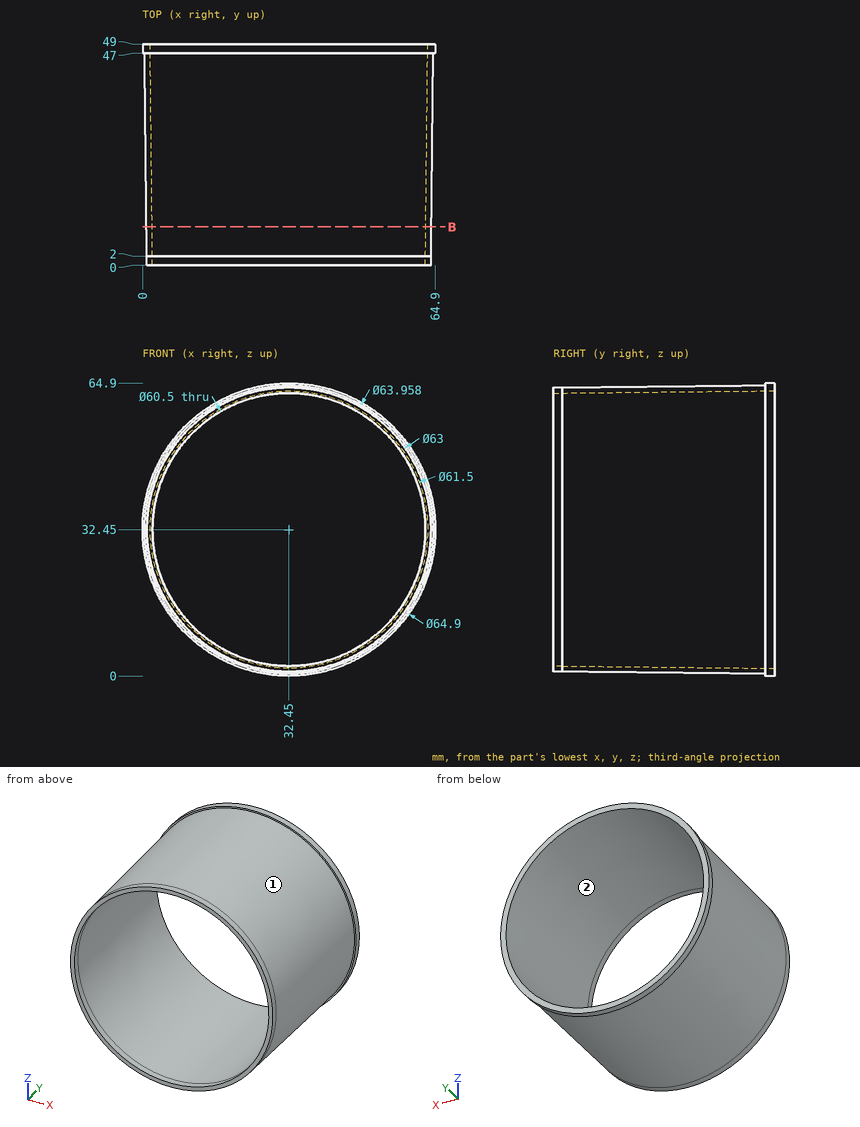
Verification items for this drawing (mm, ordinates from the low corner). Coordinates: 2 decimals unless noted, no trailing zeros. Loops run counter-clockwise (first coordinate to the right, second up) from the corner with the lowest first, then second, coordinate; pieces in that order, holes last. Notation, with made-up numbers: (-10, -13) -> (40, -13) arc R20 ccw to (40, -3) -> close; hole circle Ø1 at (89.5, 23). An arc over 180 degrees is marked (long way). Answer in a Markdown table with one row per item. Add a question column.
1. Depth check by flat-ended pin: P1, Ø2, axis at y = 41, z = 47, coming from the +X side (1 decimal); P2, Ø10, axis at y = 43, z = 57, coming from the -X side (1 decimal); P3, Ø8, axis at y = 23, z = 10, coming from the +X side; P4, Ø5, axis at x = 9.5, z = 44, coming from the +Y side. Enter the tip coordinate at first touch or a pass-through.
2. Draft check along X on the marked faces 1 and 2. Enter one of: +X half, -X half, draft (parallel to the pull), parting line (faces both ways), or undercut.
3. Section check B-B, the plane y = 8.5. Enter the section's corners in (x, z).
4. Material ranges on probe 1 along X at (y, z) = (0.7, 32.45); probe 2 along X at (y, z) = (30.5, 8) (1 decimal), recorded low to high. Write a range as [from, to].
Derived:
| question | item | result |
|---|---|---|
| 1 | P1 | stops at x = 61.3 |
| 1 | P2 | stops at x = 7.2 |
| 1 | P3 | stops at x = 58.26 |
| 1 | P4 | passes through |
| 2 | face 1 | parting line |
| 2 | face 2 | undercut |
| 3 | outline | circle Ø63.14 at (32.45, 32.45); hole circle Ø60.64 at (32.45, 32.45) |
| 4 | probe 1 | x = [0.95, 2.2], [62.7, 63.95] |
| 4 | probe 2 | x = [12.1, 14.1], [50.8, 52.8] |
